Source: CAD feature listing. Evaluate the final solid. Frame: model axes, mm. A direction names the side the tool comes from. Give positions to 0.01 mm unless a question says otherwise; leave off trailing zeros. Order: outer loops, then holes, each group sorted by start corner. A loop starts at its lowest first (then second) coordinate and runs counter-clockwise, first axis right, second up. Notation, with made-up numbers: M 7,-25 L 19,-25 A12 ccw 19,-4 Z; hole C 74.25,-31.5 d7. An arc over 180 degrees is marked long. Answer as a JSON object with one key per item and string values. Group by question number.
1. Section query A-A (y = 0). Output: boundary loops of the cut face in (x, z).
2. Section query C-C (z = 7). Output: boundary loops of the cut face in (x, y), plus the area to 3 significant figures.
3. Pin query (flat end, axial travel): P1, Ø3, axis at y = 23.5, z = 3.5, coming from the +X side; P2, Ø3, axis at x = 2.5, y = 25, coming from the +Z side; P3, Ø0.8, axis at y = -1, z = 8, coming from the +X side. Return the tip coordinate at first contact, or that it passes through.
4. Section query B-B (x = 6.75). Output: boundary loops of the cut face in (y, z).
5. Section query D-D (z = 4). Output: boundary loops of the cut face in (x, y).
6. Set-up query: faces 4 (the flat face through (3, -3, 6.35)), 5 (the flat face through (1.89, -3.33, 7.6)), 6 (the flat face through (-1.89, 3.33, 7.6)). Return all of +Z, -Z, +X, -X, +Y, -Y with unobstructed straight access to the full face (end or side cutting, diameter ignored); none if empty.
7. Pull-direction query (X, two-part tool) for faces 1 (the flat face through (3.828, 0, 8)), 2 (the flat face through (0, 10, 0)), 3 (the cylindrical face through (-0.17, 32.65, 2.5)); classes: +X half, -X half, draft (parallel to the pull), parting line (faces both ways), or undercut.
8. Material intervals for L1, parallel to Z at x = 7.25, y = 8; L2, parallel to Z at x = 0, y = -7; L3, parallel to X at y = 2, z = 7.75, sorted ascending. Write a range as [from, to].
from build123d import *

# Parameters (mm, degrees)
F2_R     = 1.27
F3_DEPTH = 5.08
F0_R     = 10.902803
F4_DEPTH = 5.08
F5_R     = 7.588096
F6_DEPTH = 1.27
F8_DEPTH = 2.54


with BuildPart() as f3:
    # F2 (on face) → F3 (new body)
    with BuildSketch(Plane.XY):
        Polygon((10.719042, 0), (0, 41.089665), (-10.719042, 0), align=None)
        with Locations((0, 31.391483)):
            Circle(F2_R, mode=Mode.SUBTRACT)
    extrude(amount=F3_DEPTH)

    # F0 (on Top) → F4 (join)
    with BuildSketch(Plane.XY):
        Circle(F0_R)
    extrude(amount=F4_DEPTH)

    # F5 (on face) → F6 (join)
    with BuildSketch(Plane.XY.offset(5.08)):
        Circle(F5_R)
    extrude(amount=F6_DEPTH)

    # F7 (on face) → F8 (join)
    with BuildSketch(Plane.XY.offset(6.35)):
        Polygon((3.828231, -2.21023), (3.828231, 2.21023), (0, 4.42046), (-3.828231, 2.21023), (-3.828231, -2.21023), (0, -4.42046), align=None)
    extrude(amount=F8_DEPTH)


solid = f3.part
Answer sheet:
{
 "1": {"outline": "M -10.9,0 L 10.9,0 L 10.9,5.08 L 7.59,5.08 L 7.59,6.35 L 3.83,6.35 L 3.83,8.89 L -3.83,8.89 L -3.83,6.35 L -7.59,6.35 L -7.59,5.08 L -10.9,5.08 Z"},
 "2": {"outline": "M -3.83,-2.21 L 0,-4.42 L 3.83,-2.21 L 3.83,2.21 L 0,4.42 L -3.83,2.21 Z", "area": "50.8 mm^2"},
 "3": {"P1": "x = 4.98", "P2": "z = 5.08", "P3": "x = 3.83"},
 "4": {"outline": "M -8.56,0 L 15.21,0 L 15.21,5.08 L 3.47,5.08 L 3.47,6.35 L -3.47,6.35 L -3.47,5.08 L -8.56,5.08 Z"},
 "5": {"outline": "M -9.19,5.87 A10.9 ccw long 9.19,5.87 L 0,41.09 Z; hole C 0,31.39 d2.54"},
 "6": {"face 4": "+Z", "face 5": "+Z, +X, -Y", "face 6": "+Z, -X, +Y"},
 "7": {"face 1": "+X half", "face 2": "draft", "face 3": "undercut"},
 "8": {"L1": "[0, 5.08]", "L2": "[0, 6.35]", "L3": "[-3.83, 3.83]"}
}
